The listing builds one solid part. Answer for the finished solid, in the listing's coordinates (mm). Face numbers are marked on the shaded views. Give positions to 0.01 mm unless a question says otherwise; leave off trailing zeros. Order: outer loops, then holes, each group sorted by start corner. A loop starts at its lowest first (then second) coordinate and runs counter-clockwise, first axis right, second up. Notation, with made-up numbers: (17.5, -39.5) - (39.5, -39.5) arc R22 cw to (39.5, -8.5) - close; hole circle Ø7 at (13, 73). An arc over 180 degrees is marked (long way). Use a Markdown table: item, result. Add a question column.
1) Straight lines are drawn through the part: line 1 (Y direction, x = 21.5, z = 6.5); line 2 (Z direction, x = 103.5, y = 3); line 3 (Z direction, x = 111.5, y = 6.75). For each, find the intervals that lie inside material, in ascending order.
2) Find section A-A, the plane x = 9.5. Determine the outline of the cut face in (y, z), plus the area to 3 significant figures.
3) The mould has two halves that part along Y. Classify the marked faces 1, 2 and 3: released by +Y, released by -Y, zero draft, split by the parting line, or undercut.
4) Flat-ended cylindrical pins translate along their axes: pin 1 (1.5 mm diameter, centred on x = 46, z = 77.5, fed in from +Y); pin 2 (1.5 mm diameter, centred on y = 2.5, z = 95, fed in from +X); pin 3 (2 mm diameter, centred on x = 46.5, y = 5, fed in from -Z); pin 4 (1.4 mm diameter, centred on x = 68.5, y = 2.5, fed in from -Z). Find the tip coordinate at first contact, or state that the pin passes through.
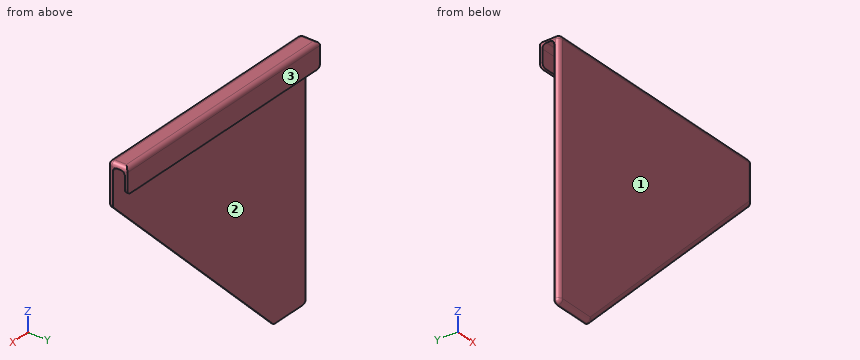
from build123d import *

# Parameters (mm, degrees)
F1_W     = 120
F1_H     = 2
F2_DEPTH = 7
F3_DEPTH = 2.54
F4_W     = 120
F4_H     = 1.2
F5_DEPTH = 10
F6_R     = 1.9999


# Not quite as in the source:
# - a fillet or chamfer is up to 0.001 mm smaller than in the source, because OpenCascade refuses the exact size


with BuildPart() as f2:
    # F1 (on face) → F2 (new body)
    with BuildSketch(Plane.XZ):
        with Locations((60, 119)):
            Rectangle(F1_W, F1_H)
    extrude(amount=-F2_DEPTH)

    # F0 (on Front) → F3 (join)
    with BuildSketch(Plane.XZ):
        Polygon((0, 120), (0, 0), (20, 0), (120, 100), (120, 120), align=None)
    extrude(amount=F3_DEPTH)

    # F4 (on face) → F5 (join)
    with BuildSketch(Plane(origin=(0, 0, 118), x_dir=(1, 0, 0), z_dir=(0, 0, -1))):
        with Locations((60, -6.4)):
            Rectangle(F4_W, F4_H)
    extrude(amount=F5_DEPTH)

    # F6 (radius 2 in the source; OpenCascade refuses exactly that, so slightly less here)
    f6_edges = [f2.edges().sort_by_distance(p)[0] for p in [
        (0, -1.27, 0),
        (20, -1.27, 0),
        (120, -1.27, 100),
        (0, 2.23, 120),
        (120, 2.23, 120),
        (120, 6.4, 108),
        (0, 6.4, 108),
        (0, -2.54, 60),
        (60, -2.54, 120),
        (120, -2.54, 110),
        (70, -2.54, 50),
        (10, -2.54, 0),
        (60, 0, 118),
        (60, 5.8, 118),
        (60, 7, 120),
    ]]
    fillet(f6_edges, radius=F6_R)


solid = f2.part
The answers:
| question | item | result |
|---|---|---|
| 1 | line 1 | -2.54 to 0 |
| 1 | line 2 | 118 to 120 |
| 1 | line 3 | 108 to 118.97 |
| 2 | outline | (-2.54, 2) arc R2 ccw to (-0.54, 0) - (0, 0) - (0, 116) arc R2 cw to (2, 118) - (3.8, 118) arc R2 cw to (5.8, 116) - (5.8, 108) - (7, 108) - (7, 118) arc R2 ccw to (5, 120) - (-0.54, 120) arc R2 ccw to (-2.54, 118) - close |
| 2 | area | 330 mm2 |
| 3 | face 1 | released by -Y |
| 3 | face 2 | undercut |
| 3 | face 3 | released by +Y |
| 4 | pin 1 | y = 0 |
| 4 | pin 2 | through |
| 4 | pin 3 | z = 108 |
| 4 | pin 4 | z = 117.99 |
